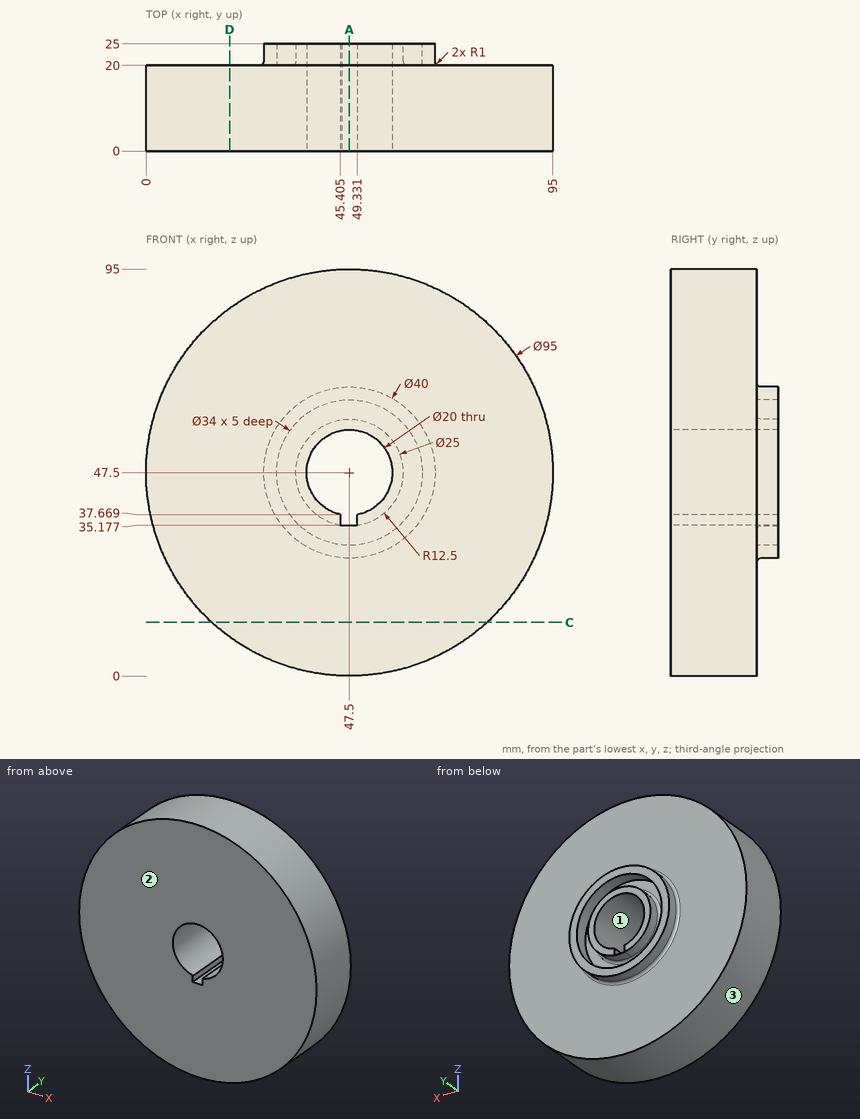
For this review, use the dimensioned drawing (mm, ordinates from the lowest corner) and the shaded views. Round coordinates to 2 decimals unless told otherwise and drop trailing zeros. Order: outer loops, then holes, each group sorted by start corner. A loop starts at its lowest first (then second) coordinate and runs counter-clockwise, first axis right, second up. Notation, with made-up numbers: (84, 71) - (91, 71) arc R22 ccw to (91, 78) - close; hole circle Ø2 at (-24.5, 57.5). An arc over 180 degrees is marked (long way). Use one line per item in the form item = value.
Q1. Add section D-D on x = 19.5. Give the boundary of the cut face in (y, z).
Response values:
outline = (0, 9.13) - (20, 9.13) - (20, 85.87) - (0, 85.87) - close
Q2. Add section A-A on x = 47.5. Give the boundary of the cut face in (y, z).
Response values:
outline = (0, 0) - (20, 0) - (20, 26.5) arc R1 cw to (21, 27.5) - (25, 27.5) - (25, 30.5) - (20, 30.5) - (20, 34) arc R1 cw to (21, 35) - (25, 35) - (25, 35.18) - (0, 35.18) - close; (0, 57.5) - (25, 57.5) - (25, 60) - (21, 60) arc R1 cw to (20, 61) - (20, 64.5) - (25, 64.5) - (25, 67.5) - (21, 67.5) arc R1 cw to (20, 68.5) - (20, 95) - (0, 95) - close
Q3. Clearance check with flat-ended pins moving along their axes: P1, Ø2, axis at x = 14, y = 20.5, coming from the +Z side (1 decimal); P2, Ø10, axis at y = 9, z = 53, coming from the -X side; P3, Ø0.7, axis at y = 15, z = 37, coming from the +X side. State where each tip first meets the part, or that it passes through.
Response values:
P1 = 82
P2 = 0
P3 = 93.9
Q4. To check wall thickness, follow line 1 (Z direction, x = 47.5, y = 22.7); line 2 (X direction, y = 20.75, z = 44) (1 decimal); line 3 (X direction, y = 20.5, z = 41.5) (1 decimal). State the ranges of each line that lie inside material, in increasing order.
Response values:
line_1 = 27.5 to 30.5, 35 to 35.18, 57.5 to 60, 64.5 to 67.5
line_2 = 27.8 to 30.9, 35.5 to 38.1, 56.9 to 59.5, 64.1 to 67.2
line_3 = 28.3 to 31.6, 36.4 to 39.5, 55.5 to 58.6, 63.4 to 66.7
Q5. Mouldability with a two-part tool opening along Z and no side actions: class the marked faces 1, 2 and 3 as pulls with the +Z half, pulls with the -Z half, needs draft (parallel to the pull), parting line crosses it, or undercut.
Response values:
face_1 = undercut
face_2 = needs draft
face_3 = parting line crosses it
Q6. Add section C-C on z = 12.5. Give the boundary of the cut face in (x, y), then the cut area to 3 significant figures.
Response values:
outline = (15.39, 0) - (79.61, 0) - (79.61, 20) - (15.39, 20) - close
area = 1,280 mm^2
